The listing builds one solid part. Answer for the finished solid, in the listing's coordinates (mm). A direction names the side the tool comes from. Coordinates: 2 decimals unless noted, no trailing zeros. Order: outer loops, then holes, each group sorted by start corner. A loop starts at its lowest first (then second) coordinate and runs counter-clockwise, first axis right, second up. Notation, with made-up numbers: M -9.75,12 L 32.25,12 A7 cw 32.25,20 Z; hole C 48,62.5 d9. An arc over 180 degrees is marked long. One line per item, written item: value. Start each with the question number.
Q1. The part is cut by section B-B on y = 0. Give the vertices of the cut face in (x, z) (3 decimals), then the cut area to 3 significant figures.
Q2. Straight lines are drawn through the part: line 1 along Y through (x, z) = (1.25, 1.5); line 2 along Y through (x, z) = (0.79, 2.1); line 3 along Z through (x, y) = (3.5, 3). For each, find the intervals that lie inside material, in ascending order. Write a range as [from, to].
Q3. For faces 1 (the flat face through (-5, 0, 3)), 2 (the flat face through (0, -4, 6)), determine the directions among +Z, -Z, +X, -X, +Y, -Y from which every point of the face is accessible in a straight line to the end or side of a thin tool.
Q4. The part is cut by section A-A on z = 1.25. Give the vertices of the cut face in (x, y).
Q5. Determine the mould class of faces 3 (the flat face through (4.7, 0, 3)), 4 (the flat face through (2.465, -4.35, 2.959)), 5 (the flat face through (-2, 0, 8.5)) for opening direction Y: pulls with the +Y half, pulls with the -Y half, needs draft (parallel to the pull), parting line crosses it, or undercut.
Q6. The part is cut by section D-D on x = 3.75. Give the vertices of the cut face in (y, z).
Q7. This flat-tipped pin is pushed along its axis until it touches: pin 1 Ø4.5 at (x, y) = (0.79, 0) entering from +Z. Where does it stop, or does it pass through?
Q8. The part is cut by section C-C on y = 4.5. Give the vertices of the cut face in (x, z).
```python
from build123d import *

# Parameters (mm, degrees)
F1_DEPTH = 6
F2_R     = 3.555
F2_R_2   = 2.5
F3_DEPTH = 2.5
F4_W     = 0.3
F4_H     = 2
F5_DEPTH = 25
F6_R     = 2.5
F7_DEPTH = 25
F8_SIZE  = 0.1


with BuildPart() as f1:
    # F0 (on Top) → F1 (new body)
    with BuildSketch(Plane.XY):
        Polygon((5, -2.886751), (5, 2.886751), (0, 5.773503), (-5, 2.886751), (-5, -2.886751), (0, -5.773503), align=None)
    extrude(amount=F1_DEPTH)

    # F2 (on face) → F3 (join)
    with BuildSketch(Plane.XY.offset(6)):
        Circle(F2_R)
        with Locations((0.79, 0)):
            Circle(F2_R_2, mode=Mode.SUBTRACT)
    extrude(amount=F3_DEPTH)

    # F4 (on face) → F5 (cut)
    with BuildSketch(Plane.XY.offset(6)):
        with Locations((4.85, 0)):
            Rectangle(F4_W, F4_H)
    extrude(amount=-F5_DEPTH, mode=Mode.SUBTRACT)

    # F6 (on face) → F7 (cut)
    with BuildSketch(Plane.XY.offset(6)):
        with Locations((0.79, 0)):
            Circle(F6_R)
    extrude(amount=-F7_DEPTH, mode=Mode.SUBTRACT)

    # F8
    f8_edges = [f1.edges().sort_by_distance(p)[0] for p in [
        (-2.5, -4.330127, 6),
        (2.5, -4.330127, 6),
        (5, -1.943376, 6),
        (5, 1.943376, 6),
        (4.7, 0, 6),
        (4.85, -1, 6),
        (4.85, 1, 6),
        (2.5, 4.330127, 6),
        (-2.5, 4.330127, 6),
        (-5, 0, 6),
        (-3.555, 0, 8.5),
        (-1.71, 0, 8.5),
        (2.5, -4.330127, 0),
        (-2.5, -4.330127, 0),
        (5, -1.943376, 0),
        (-5, 0, 0),
        (4.85, -1, 0),
        (-2.5, 4.330127, 0),
        (4.7, 0, 0),
        (2.5, 4.330127, 0),
        (4.85, 1, 0),
        (5, 1.943376, 0),
        (-1.71, 0, 0),
    ]]
    chamfer(f8_edges, length=F8_SIZE)


solid = f1.part
```
Output:
1. outline: M -5,0.1 L -4.9,0 L -1.81,0 L -1.71,0.1 L -1.71,8.4 L -1.81,8.5 L -3.455,8.5 L -3.555,8.4 L -3.555,6 L -4.9,6 L -5,5.9 Z; M 3.29,0.1 L 3.39,0 L 4.6,0 L 4.7,0.1 L 4.7,5.9 L 4.6,6 L 3.555,6 L 3.555,8.4 L 3.455,8.5 L 3.39,8.5 L 3.29,8.4 Z
1. area: 33.4 mm^2
2. line 1: y = [-5.05, -2.46], [2.46, 5.05]
2. line 2: y = [-5.32, -2.5], [2.5, 5.32]
2. line 3: z = [0, 6]
3. face 1: +Z, -Z, -X, +Y, -Y
3. face 2: +Z
4. outline: M -5,-2.89 L 0,-5.77 L 5,-2.89 L 5,-1 L 4.7,-1 L 4.7,1 L 5,1 L 5,2.89 L 0,5.77 L -5,2.89 Z; hole C 0.79,0 d5
5. face 3: undercut
5. face 4: pulls with the -Y half
5. face 5: needs draft
6. outline: M -3.61,0.1 L -3.49,0 L 3.49,0 L 3.61,0.1 L 3.61,5.9 L 3.49,6 L -3.49,6 L -3.61,5.9 Z
7. pin 1: passes through
8. outline: M -2.21,0.1 L -2.01,0 L 2.01,0 L 2.21,0.1 L 2.21,5.9 L 2.01,6 L -2.01,6 L -2.21,5.9 Z
